Design review of the part built by this model. Coordinates are the model's own, in mm. Round coordinates to 2 decimals unless told otherwise and drop trailing zeros. Loops run counter-clockwise (first coordinate to the right, second up) from the corner with the lowest first, then second, coordinate; pieces in that order, holes last. Notation, with made-up numbers: (73.25, -27) - (110.25, -27) arc R18 cw to (110.25, -16) - close; hole circle Ø4 at (28, 55.5). An arc over 180 degrees is marked (long way). Answer as CSV lines item,"result". Start each with the question number.
(1) Consider section C-C (z = 20.25). Give the boundary of the cut face in (x, y).
(2) For P1, Ø14.5, axis at x = 48.06, y = 97, coming from the +Z side, flat-tipped, find the tip position at first contact; note if it passes through.
(3) Wall thickness on L1, parallel to Y at x = 302, z = 17.25; L2, parallel to X at y = 104, z = 2; L3, parallel to Y at x = 309.5, z = 23.75: over which ranges is each line inside the solid? List them lowest first.
(4) Mouldability with a two-part tool opening along X and no side actions: class faces 1 (the cylindrical face through (2.85, 3.01, 12.68)), 2 (the cylindrical face through (310.667, 99.748, 12.325)), 3 (the cylindrical face through (346.99, 197.15, 12.68)), 4 (the flat face through (173, 101, 25)) as released by +X, released by -X, zero draft, split by the parting line, or undercut.
(5) Consider section A-A (y = 180). Give the boundary of the cut face in (x, z), and give its area (4 significant figures).
(6) Consider section B-B (x = 48). Give the boundary of the cut face in (y, z).
from build123d import *

# Parameters (mm, degrees)
F0_R     = 9.15
F1_DEPTH = 25
F2_R     = 10


with BuildPart() as f1:
    # F0 (on Top) → F1 (new body)
    with BuildSketch(Plane.XY):
        Polygon((175, 200), (0, 200), (0, 0), (350, 0), (350, 200), align=None)
        with Locations((48.060222, 97.000022)):
            Circle(F0_R, mode=Mode.SUBTRACT)
        with Locations((301.939778, 97.000022)):
            Circle(F0_R, mode=Mode.SUBTRACT)
        with Locations((48, 180)):
            Circle(F0_R, mode=Mode.SUBTRACT)
        with Locations((302, 180)):
            Circle(F0_R, mode=Mode.SUBTRACT)
    extrude(amount=F1_DEPTH)

    # F2
    f2_edges = [f1.edges().sort_by_distance(p)[0] for p in [
        (350, 0, 12.5),
        (350, 200, 12.5),
        (0, 0, 12.5),
        (0, 200, 12.5),
    ]]
    fillet(f2_edges, radius=F2_R)


solid = f1.part
Determined:
1,outline,"(0, 10) arc R10 ccw to (10, 0) - (340, 0) arc R10 ccw to (350, 10) - (350, 190) arc R10 ccw to (340, 200) - (10, 200) arc R10 ccw to (0, 190) - close; hole circle Ø18.3 at (48, 180); hole circle Ø18.3 at (48.06, 97); hole circle Ø18.3 at (301.94, 97); hole circle Ø18.3 at (302, 180)"
2,P1,"passes through"
3,L1,"y = 0 to 87.85, 106.15 to 170.85, 189.15 to 200"
3,L2,"x = 0 to 42.17, 53.95 to 296.05, 307.83 to 350"
3,L3,"y = 0 to 91.85, 102.15 to 174.76, 185.24 to 200"
4,face 1,"released by -X"
4,face 2,"undercut"
4,face 3,"released by +X"
4,face 4,"zero draft"
5,outline,"(0, 0) - (38.85, 0) - (38.85, 25) - (0, 25) - close; (57.15, 0) - (292.85, 0) - (292.85, 25) - (57.15, 25) - close; (311.15, 0) - (350, 0) - (350, 25) - (311.15, 25) - close"
5,area,"7,835 mm^2"
6,outline,"(0, 0) - (87.85, 0) - (87.85, 25) - (0, 25) - close; (106.15, 0) - (170.85, 0) - (170.85, 25) - (106.15, 25) - close; (189.15, 0) - (200, 0) - (200, 25) - (189.15, 25) - close"
